```python
from build123d import *

# Parameters (mm, degrees)
SKETCH_1_R          = 4.4
EXTRUDE_1_DEPTH     = 0.7
SKETCH_2_R          = 3.35
EXTRUDE_2_DEPTH     = 1
SKETCH_3_R          = 3.4
EXTRUDE_3_DEPTH     = 3.9
SKETCH_4_R          = 10.526345736
SKETCH_4_R_2        = 3.3
CUT_EXTRUDE_1_DEPTH = 1
CUT_EXTRUDE_2_DEPTH = 2
SKETCH_6_R          = 2
EXTRUDE_4_DEPTH     = 5


with BuildPart() as part:
    # 草图1 → 凸台-拉伸1 (new body)
    with BuildSketch(Plane(origin=(0, 0, 0), x_dir=(1, 0, 0), z_dir=(0, 1, 0))):
        Circle(SKETCH_1_R)
    extrude(amount=EXTRUDE_1_DEPTH)

    # 草图2 → 凸台-拉伸2 (add)
    with BuildSketch(Plane(origin=(0, 0.7, 0), x_dir=(1, 0, 0), z_dir=(0, 1, 0))):
        Circle(SKETCH_2_R)
    extrude(amount=EXTRUDE_2_DEPTH)

    # 草图3 → 凸台-拉伸3 (add)
    with BuildSketch(Plane(origin=(0, 1.7, 0), x_dir=(1, 0, 0), z_dir=(0, 1, 0))):
        Circle(SKETCH_3_R)
    extrude(amount=EXTRUDE_3_DEPTH)

    # 草图4 → 切除-拉伸1 (cut)
    with BuildSketch(Plane.XZ.offset(-1.7)):
        Circle(SKETCH_4_R)
        Circle(SKETCH_4_R_2, mode=Mode.SUBTRACT)
    extrude(amount=-CUT_EXTRUDE_1_DEPTH, mode=Mode.SUBTRACT)

    # 草图5 → 切除-拉伸2 (cut)
    with BuildSketch(Plane(origin=(0, 5.6, 0), x_dir=(1, 0, 0), z_dir=(0, 1, 0))):
        Polygon((-1.729316128, 0), (-0.864658064, -1.497631698), (0.864658064, -1.497631698), (1.729316128, 0), (0.864658064, 1.497631698), (-0.864658064, 1.497631698), align=None)
    extrude(amount=-CUT_EXTRUDE_2_DEPTH, mode=Mode.SUBTRACT)

    # 草图6 → 凸台-拉伸4 (add)
    with BuildSketch(Plane.XZ):
        Circle(SKETCH_6_R)
    extrude(amount=EXTRUDE_4_DEPTH)


solid = part.part
```
Model file for the job. Use its own axes, mm. A direction names the side the tool comes from. Coordinates: 2 decimals unless noted, no trailing zeros. Loops run counter-clockwise (first coordinate to the right, second up) from the corner with the lowest first, then second, coordinate; pieces in that order, holes last. Notation, with made-up numbers: (71.25, 23) - (119.25, 23) arc R19 cw to (119.25, 51) - close; hole circle Ø7 at (33, 76.5). An arc over 180 degrees is marked (long way). Write item = value, one per line. Start each with the question number.
Item 1: Drop flat-ended pins along their axis: pin 1 Ø4 at (y, z) = (0, 3) entering from -X; pin 2 Ø0.5 at (x, y) = (0, 5) entering from +Z; pin 3 Ø1 at (x, y) = (3.5, 3.5) entering from +Z. Give the stop position or say it passes through.
Item 2: Saw through at A-A, the plane y = 5. List the corners of the cut face in (x, z), then the cut area to 3 significant figures.
Item 3: Wall check: probe 1 along Z at (x, y) = (0, 3.75); probe 2 along Z at (x, y) = (0, 1.75); probe 3 along Y at (x, z) = (-0.25, -3). Give the ranges that are in metal, low to high. Write a range as [from, to].
Item 4: Saw through at C-C, the plane z = 0.25. List the corners of the cut face in (x, y).
Item 5: 3-axis set-ups, long thin cutter, end or side, ignore diameter. For faces 4 (the face through (-2.43, 2.19, 2.23)), 5 (the face through (0, -2, -2)), 6 (the face through (0, 3.6, 0)): which of +Z, -Z, +X, -X, +Y, -Y reach the whole face in a straight line?
Item 6: Saw through at B-B, the plane x = 0. List the corners of the cut face in (y, z), then the cut area to 3 significant figures.
Item 7: Saw through at D-D, the plane y = 2.5. List the corners of the cut face in (x, z), then the cut area to 3 significant figures.
Item 8: Pull direction Y, two halves, no side cores. Call faces 1 (the face through (-3.347, 1.193, -0.147)), 2 (the face through (2, 0, 1)), 3 (the face through (1.29, 4.61, 0.76)): +Y half, -Y half, draft (parallel to the pull), parting line (faces both ways), or undercut.
Answers:
q1.pin_1 = -4.28
q1.pin_2 = 3.4
q1.pin_3 = 1.6
q2.outline = circle Ø6.8 at (0, 0); hole (-1.73, 0) - (-0.86, -1.5) - (0.86, -1.5) - (1.73, 0) - (0.86, 1.5) - (-0.86, 1.5) - close
q2.area = 28.5 mm2
q3.probe_1 = [-3.4, -1.5], [1.5, 3.4]
q3.probe_2 = [-3.3, 3.3]
q3.probe_3 = [0, 5.6]
q4.outline = (-4.39, 0) - (-1.98, 0) - (-1.98, -5) - (1.98, -5) - (1.98, 0) - (4.39, 0) - (4.39, 0.7) - (3.34, 0.7) - (3.34, 1.7) - (3.29, 1.7) - (3.29, 2.7) - (3.39, 2.7) - (3.39, 5.6) - (1.58, 5.6) - (1.58, 3.6) - (-1.58, 3.6) - (-1.58, 5.6) - (-3.39, 5.6) - (-3.39, 2.7) - (-3.29, 2.7) - (-3.29, 1.7) - (-3.34, 1.7) - (-3.34, 0.7) - (-4.39, 0.7) - close
q5.face_4 = none
q5.face_5 = -Y
q5.face_6 = +Y
q6.outline = (-5, -2) - (0, -2) - (0, -4.4) - (0.7, -4.4) - (0.7, -3.35) - (1.7, -3.35) - (1.7, -3.3) - (2.7, -3.3) - (2.7, -3.4) - (5.6, -3.4) - (5.6, -1.5) - (3.6, -1.5) - (3.6, 1.5) - (5.6, 1.5) - (5.6, 3.4) - (2.7, 3.4) - (2.7, 3.3) - (1.7, 3.3) - (1.7, 3.35) - (0.7, 3.35) - (0.7, 4.4) - (0, 4.4) - (0, 2) - (-5, 2) - close
q6.area = 53.2 mm2
q7.outline = circle Ø6.6 at (0, 0)
q7.area = 34.2 mm2
q8.face_1 = undercut
q8.face_2 = -Y half
q8.face_3 = draft
